```python
from build123d import *

# Parameters (mm, degrees)
F0_W     = 304.8
F0_H     = 203.2
F1_DEPTH = 19.05
F2_SIZE  = 50.8
F3_W     = 228.6
F3_H     = 25.4
F4_DEPTH = 19.05
F5_R     = 6.35
F7_D     = 12.7
F7_DEPTH = 12.7
F7_TIP   = 3.8154649308
F8_D     = 12.7
F8_DEPTH = 12.7
F8_TIP   = 3.8154649308
F9_D     = 9.525


with BuildPart() as f1:
    # F0 (on Front) → F1 (new body)
    with BuildSketch(Plane.XZ):
        with Locations((139.2554994464, 77.2159987301)):
            Rectangle(F0_W, F0_H)
    extrude(amount=F1_DEPTH)

    # F2
    f2_edges = [f1.edges().sort_by_distance(p)[0] for p in [
        (-13.144501, -9.525, 178.815999),
        (291.655499, -9.525, 178.815999),
    ]]
    chamfer(f2_edges, length=F2_SIZE)

    # F3 (on face) → F4 (cut)
    with BuildSketch(Plane.XZ.offset(19.05)):
        with Locations((139.2554994464, -11.6840012699)):
            Rectangle(F3_W, F3_H)
    extrude(amount=-F4_DEPTH, mode=Mode.SUBTRACT)

    # F5
    f5_edges = [f1.edges().sort_by_distance(p)[0] for p in [
        (24.955499, -9.525, 1.015999),
        (253.555499, -9.525, 1.015999),
        (253.555499, -9.525, -24.384001),
        (291.655499, -9.525, -24.384001),
        (24.955499, -9.525, -24.384001),
        (-13.144501, -9.525, -24.384001),
    ]]
    fillet(f5_edges, radius=F5_R)

    # F7
    with Locations(Plane.XZ.offset(19.05)):
        with Locations((12.2554994464, 109.8041987301), (266.2554994464, 109.8041987301)):
            Hole(F7_D / 2, depth=F7_DEPTH)
            with Locations((0, 0, -(F7_DEPTH + F7_TIP / 2))):  # 118° drill point
                Cone(0, F7_D / 2, F7_TIP, mode=Mode.SUBTRACT)

    # F8
    with Locations(Plane.XZ.offset(19.05)):
        with Locations((272.6054994464, 70.8659987301), (5.9054994464, 70.8659987301), (5.9054994464, -5.3340012699), (272.6054994464, -5.3340012699)):
            Hole(F8_D / 2, depth=F8_DEPTH)
            with Locations((0, 0, -(F8_DEPTH + F8_TIP / 2))):  # 118° drill point
                Cone(0, F8_D / 2, F8_TIP, mode=Mode.SUBTRACT)

    # F9 (through all)
    with Locations(Plane.XZ.offset(19.05)):
        with Locations((5.9054994464, 70.8659987301), (272.6054994464, 70.8659987301), (5.9054994464, -5.3340012699), (272.6054994464, -5.3340012699)):
            Hole(F9_D / 2)


solid = f1.part
```
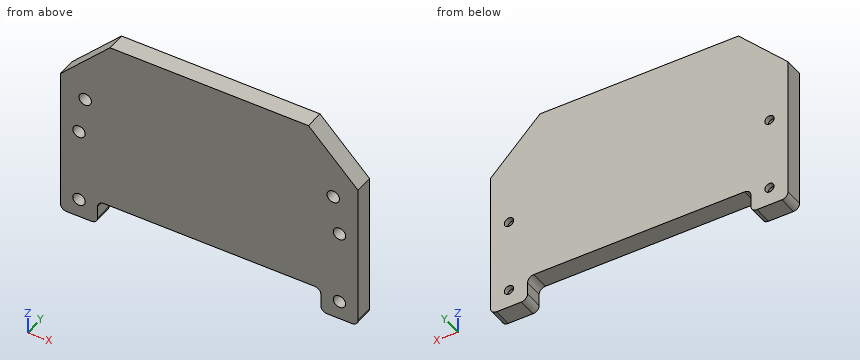
Input: part model. Units: mm. Frame: model coordinates. Coordinates: 2 decimals unless noted, no trailing zeros. Loops run counter-clockwise (first coordinate to the right, second up) from the corner with the lowest first, then second, coordinate; pieces in that order, holes last.
Q1. Section B-B, the plane x = 109. Return the cut outline in (y, z).
Results are:
outline: (-19.05, 1.02) - (0, 1.02) - (0, 178.82) - (-19.05, 178.82) - close
Q2. Section C-C, the plane z = 132. Return the cut outline in (x, y).
Results are:
outline: (-9.16, -19.05) - (287.67, -19.05) - (287.67, 0) - (-9.16, 0) - close
Q3. Line query: line 1 along X through (y, z) = (-1.25, -11); line 2 along Z through (x, y) = (119, -9); line 3 along X through (y, z) = (-7.5, -3). Output: solid intervals per line, ascending.
Results are:
line 1: x = -13.14 to 24.96, 253.56 to 291.66
line 2: z = 1.02 to 178.82
line 3: x = -13.14 to 0, 11.81 to 25.4, 253.11 to 266.7, 278.51 to 291.66
Q4. Contact query for flat-ended pins moving along their axis: pin 1 (4 mm diameter, centred on x = 222.5, z = 83, fed in from +Y); pin 2 (11.5 mm diameter, centred on x = 5.91, z = -5.33, fed in from -Y); pin 3 (8.5 mm diameter, centred on x = 5.91, z = -5.33, fed in from +Y); pin 4 (11 mm diameter, centred on x = 272.61, z = -5.33, fed in from -Y). Output: stop coordinate, or through.
Results are:
pin 1: stops at y = 0
pin 2: stops at y = -5.99
pin 3: passes through
pin 4: stops at y = -5.84
Q5. Section A-A, the plane y = -10.25. Return the cut outline in (x, z).
Results are:
outline: (-13.14, -18.03) arc R6.35 ccw to (-6.79, -24.38) - (18.61, -24.38) arc R6.35 ccw to (24.96, -18.03) - (24.96, -5.33) arc R6.35 cw to (31.31, 1.02) - (247.21, 1.02) arc R6.35 cw to (253.56, -5.33) - (253.56, -18.03) arc R6.35 ccw to (259.91, -24.38) - (285.31, -24.38) arc R6.35 ccw to (291.66, -18.03) - (291.66, 128.02) - (240.86, 178.82) - (37.66, 178.82) - (-13.14, 128.02) - close; hole circle Ø12.7 at (5.91, -5.33); hole circle Ø12.7 at (5.91, 70.87); hole circle Ø12.7 at (12.26, 109.8); hole circle Ø12.7 at (266.26, 109.8); hole circle Ø12.7 at (272.61, -5.33); hole circle Ø12.7 at (272.61, 70.87)
